from build123d import *

# Parameters (mm, degrees)
FILLET1_R = 0.75


with BuildPart() as part:
    # Sketch1 → Revolve1 (revolve)
    with BuildSketch(Plane.XY, mode=Mode.PRIVATE) as revolve1_sk:
        Polygon((0, 7.5), (-7.75, 6.018214298), (-7.75, 4.518214298), (-6.927372109, 4.518214298), (-6.927372109, 2.927787826), (-7.75, 2.927787826), (-7.75, 1.427787826), (-6.927372109, 1.427787826), (-6.927372109, 0), (-5.136257755, 0), (-3.126714823, 1.427787826), (-3.126714823, 4.7), (0, 4.7), align=None)
    revolve(revolve1_sk.sketch.rotate(Axis((0, 0, 0), (0, 1, 0)), 270), axis=Axis((0, 0, 0), (0, 1, 0)))

    # Fillet1
    fillet1_edges = [part.edges().sort_by_distance(p)[0] for p in [
        (0, 6.018214298, 7.75),
        (0, 4.518214298, 7.75),
        (0, 2.927787826, 7.75),
        (0, 1.427787826, 7.75),
    ]]
    fillet(fillet1_edges, radius=FILLET1_R - 0.0001)  # a hair under: the kernel refuses the full size


solid = part.part
Verification items for the finished model (mm, model axes). A direction names the side the tool comes from. Coordinates: 2 decimals unless noted, no trailing zeros. Order: outer loops, then holes, each group sorted by start corner. A loop starts at its lowest first (then second) coordinate and runs counter-clockwise, first axis right, second up.
Item 1: Depth check by flat-ended pin: pin 1 (1 mm diameter, centred on x = -2.5, z = -0.5, fed in from -Y); pin 2 (1.5 mm diameter, centred on x = 5, z = 1, fed in from +Y); pin 3 (1.5 mm diameter, centred on x = -2.5, y = 1, fed in from +Z). Enter the tip coordinate at first touch or a pass-through.
Filled in:
pin 1: stops at y = 4.7
pin 2: stops at y = 6.67
pin 3: stops at z = 7.24
Item 2: Section check A-A, the plane y = 6.5. Enter the section's corners in (x, z).
Filled in:
outline: circle Ø10.46 at (0, 0)
Item 3: Access from +Z, -Z, +X, -X, +Y, -Y to the whole of each face (thin tool, end or side, straight path). Record for faces 4 (the face through (6.763, 0.704, 1.502)), 5 (the face through (-0.134, 7.415, -0.426)).
Filled in:
face 4: -Y
face 5: +Y
Item 4: Release check for a two-part mould opening along Z. For faces 1 (the face through (0, 4.7, 0)), 2 (the face through (3, 0, 5)), 3 (the face through (6.763, 3.712, 1.502)) record: +Z half, -Z half, draft (parallel to the pull), parting line (faces both ways), or undercut.
Filled in:
face 1: undercut
face 2: draft
face 3: parting line
Item 5: Material ranges on L1, parallel to X at y = 3.9, z = 0; L2, parallel to Y at x = -2, z = -2.25; L3, parallel to Y at x = 4.75, z = 5.5, recorded low to high.
Filled in:
L1: x = -6.93 to -3.13, 3.13 to 6.93
L2: y = 4.7 to 6.92
L3: y = 1.48 to 2.88, 4.57 to 6.1
